For this review, take the finished solid that the model builds, in its own axes (mm). Give positions to 0.01 mm unless a question says otherwise; leave off trailing zeros. Write each loop counter-clockwise with the first axis right and the second up, starting at its lowest first coordinate (ties: lowest second). Pieces come first, ordered by that corner, then holes. Notation, with made-up numbers: (77.5, 3.25) -> (83.5, 3.25) arc R32 cw to (83.5, 34.25) -> close; hole circle Ø2 at (-22, 59.25). An arc over 180 degrees is marked (long way). Return JSON: item names as keys, results as strings.
Autodesk Inventor part; units mm, degrees
ref_plane "Work Plane1" through (0, 1.5, 0) normal (0, 1, 0) x (1, 0, 0)
ref_plane "YZ Plane" through (0, 0, 0) normal (1, 0, 0) x (0, 1, 0)
ref_plane "XZ Plane" through (0, 0, 0) normal (0, 1, 0) x (-1, 0, 0)
sketch "Sketch1" plane through (0, 0, 0) normal (0, 1, 0) x (-1, 0, 0)
  circle A0 centre (0, 0) radius 5
  circle A1 centre (-25.7936, 17.1957) radius 5
  line L0 (-4.715, -1.6641) -> (-25.5162, 12.2034)
  line L1 (-0.2774, 4.9923) -> (-21.0786, 18.8598)
  line L2 (0, 0) -> (-25.7936, 0) construction
  line L3 (-25.7936, 0) -> (-25.7936, 17.1957) construction
  line L4 (0, 0) -> (-25.7936, 17.1957) construction
  dimension "d0" = 10
  dimension "d1" = 10
  dimension "d2" = 4
  dimension "d3" = 4
  dimension "d27" = 25
  dimension "d28" = 33.69
extrude "Extrusion1" add sketch "Sketch1" along normal blind 5
sketch "Sketch2" plane through (0, 0, 0) normal (0, -1, 0) x (1, 0, 0)
  line L0 (0, 0) -> (25.7936, 17.1957) construction
  arc A0 (25.5162, 12.2034) -> (21.0786, 18.8598) centre (25.7936, 17.1957) ccw
  line L1 (0.2774, 4.9923) -> (21.0786, 18.8598)
  arc A1 (0.2774, 4.9923) -> (4.715, -1.6641) centre (0, 0) ccw
  line L2 (25.5162, 12.2034) -> (4.715, -1.6641)
hole "Hole1" at (25.7936, 0, 17.1957) direction (0, 1, 0) diameter 3.1 end through all
ref_plane "Work Plane1" through (0, 1.5, 0) normal (0, 1, 0) x (1, 0, 0)
sketch "Sketch4" plane through (0, 5, 0) normal (0, 1, 0) x (1, 0, 0)
  circle A0 centre (25.7936, -17.1957) radius 1.55
  arc A1 (21.0786, -18.8598) -> (25.5162, -12.2034) centre (25.7936, -17.1957) ccw
  line L0 (25.5162, -12.2034) -> (4.715, 1.6641)
  arc A2 (4.715, 1.6641) -> (0.2774, -4.9923) centre (0, 0) ccw
  line L1 (0.2774, -4.9923) -> (21.0786, -18.8598)
hole "Hole2" at (0, 5, 0) direction (0, -1, 0) diameter 2.459 end through all
properties part number "gripper_hand_connector"
1. To check wall thickness, follow probe 1 along Z at (x, y) = (0, 3.7); probe 2 along X at (y, z) = (0.35, 16.5); probe 3 along X at (y, z) = (3.9, 0). State the ranges of each line that lie inside material, in increasing order.
Results found:
{"probe 1": "z = -5 to -1.23, 1.23 to 5", "probe 2": "x = 17.54 to 24.41, 27.18 to 30.74", "probe 3": "x = -5 to -1.23, 1.23 to 7.21"}
2. Add section C-C, the plane x = 28. State the section outline as (y, z) points.
Results found:
{"outline": "(0, 12.71) -> (5, 12.71) -> (5, 21.68) -> (0, 21.68) -> close"}
3. For pin 1 (12 mm diameter, centred on x = 14.5, z = 1.5, fed in from -Y); pin 2 (3 mm diameter, centred on y = 1.5, z = 3, fed in from -X); pin 3 (2 mm diameter, centred on x = 7, y = 2, fed in from +Z), all flat-tipped, find the tip position at first contact; note any pin that passes through.
Results found:
{"pin 1": "stops at y = 0", "pin 2": "stops at x = -4.77", "pin 3": "stops at z = 10.14"}
4. The part is to be moulded in two halves that separate along X. For faces 1 (the cylindrical face through (0.748, 2.465, -0.976)), 2 (the flat face through (10.532, 2.465, 11.829)), 3 (the cylindrical face through (25.725, 2.535, 18.744)), 4 (the flat face through (13, 5, 9)), say which applies: +X half, -X half, draft (parallel to the pull), parting line (faces both ways), or undercut.
Results found:
{"face 1": "undercut", "face 2": "-X half", "face 3": "undercut", "face 4": "draft"}
5. Add section B-B, the plane y = 3.75. Count the separate pieces of the cut face and the enclosed holes in it, plus the area to 3 significant figures.
Results found:
{"separate pieces": "1", "enclosed holes": "2", "area": "322 mm²"}
6. Add section A-A, the plane z = 16.5. State the section outline as (x, y) points.
Results found:
{"outline": "(17.54, 0) -> (24.41, 0) -> (24.41, 5) -> (17.54, 5) -> close; (27.18, 0) -> (30.74, 0) -> (30.74, 5) -> (27.18, 5) -> close"}
7. Add section D-D, the plane z = 0. State the section outline as (x, y) points.
Results found:
{"outline": "(-5, 0) -> (-1.23, 0) -> (-1.23, 5) -> (-5, 5) -> close; (1.23, 0) -> (7.21, 0) -> (7.21, 5) -> (1.23, 5) -> close"}
